Source: CAD feature listing. Evaluate the final solid. Frame: model axes, mm. A direction names the side the tool comes from. Coordinates: 2 decimals unless noted, no trailing zeros. Loops run counter-clockwise (first coordinate to the right, second up) from the corner with the lowest first, then second, coordinate; pieces in that order, holes last.
```python
from build123d import *

# Parameters (mm, degrees)
SKETCH1_R           = 23.8125
SKETCH1_R_2         = 10.4775
SKETCH1_R_3         = 1.905
BOSS_EXTRUDE1_DEPTH = 3.683


with BuildPart() as part:
    # Sketch1 → Boss-Extrude1 (new body)
    with BuildSketch(Plane(origin=(0, 0, 0), x_dir=(1, 0, 0), z_dir=(0, 1, 0))):
        with BuildLine():
            Line((-8.06473402, -4.72806869), (-8.06473402, 14.671308994))
            ThreePointArc((-8.06473402, 14.671308994), (-9.661605647, 23.535341917), (-14.251433206, 31.284829748))
            Line((-14.251433206, 31.284829748), (-39.858713959, 60.899286273))
            ThreePointArc((-39.858713959, 60.899286273), (-38.889761495, 87.184032671), (-12.602664438, 88.086967018))
            Line((-12.602664438, 88.086967018), (16.963304526, 62.391553913))
            ThreePointArc((16.963304526, 62.391553913), (24.731110608, 57.771090259), (33.625027761, 56.16306869))
            Line((33.625027761, 56.16306869), (53.14973402, 56.16306869))
            ThreePointArc((53.14973402, 56.16306869), (55.39479805, 55.23313272), (56.32473402, 52.98806869))
            Line((56.32473402, 52.98806869), (56.32473402, -4.72806869))
            ThreePointArc((56.32473402, -4.72806869), (55.39479805, -6.97313272), (53.14973402, -7.90306869))
            Line((53.14973402, -7.90306869), (-4.88973402, -7.90306869))
            ThreePointArc((-4.88973402, -7.90306869), (-7.13479805, -6.97313272), (-8.06473402, -4.72806869))
        make_face()
        with Locations(Location((24.13, 24.13, 0), (0, 0, 270))):
            Circle(SKETCH1_R, mode=Mode.SUBTRACT)
        with Locations(Location((-25.261408666, 73.521408666, 0), (0, 0, 270))):
            Circle(SKETCH1_R_2, mode=Mode.SUBTRACT)
        with Locations(Location((-36.294042469, 84.309426168, 0), (0, 0, 270))):
            Circle(SKETCH1_R_3, mode=Mode.SUBTRACT)
        with Locations(Location((-29.421941059, 88.38042278, 0), (0, 0, 270))):
            Circle(SKETCH1_R_3, mode=Mode.SUBTRACT)
        with Locations(Location((-10.402394551, 77.681941059, 0), (0, 0, 270))):
            Circle(SKETCH1_R_3, mode=Mode.SUBTRACT)
        with Locations(Location((-10.312858771, 69.695028354, 0), (0, 0, 270))):
            Circle(SKETCH1_R_3, mode=Mode.SUBTRACT)
        with Locations(Location((-29.087788977, 58.572858771, 0), (0, 0, 270))):
            Circle(SKETCH1_R_3, mode=Mode.SUBTRACT)
        with Locations(Location((-36.049426168, 62.488774863, 0), (0, 0, 270))):
            Circle(SKETCH1_R_3, mode=Mode.SUBTRACT)
        with BuildLine():
            ThreePointArc((44.60009114, -5.905215683), (49.831544821, -1.571544821), (54.165215683, 3.65990886))
            ThreePointArc((54.165215683, 3.65990886), (53.580347261, 6.748102738), (50.492153383, 6.163234317))
            ThreePointArc((50.492153383, 6.163234317), (46.688455179, 1.571544821), (42.096765683, -2.232153383))
            ThreePointArc((42.096765683, -2.232153383), (41.511897262, -5.320347261), (44.60009114, -5.905215683))
        make_face(mode=Mode.SUBTRACT)
        with BuildLine():
            ThreePointArc((44.60009114, 54.165215683), (49.831544821, 49.831544821), (54.165215683, 44.60009114))
            ThreePointArc((54.165215683, 44.60009114), (53.580347261, 41.511897262), (50.492153383, 42.096765683))
            ThreePointArc((50.492153383, 42.096765683), (46.688455179, 46.688455179), (42.096765683, 50.492153383))
            ThreePointArc((42.096765683, 50.492153383), (41.511897262, 53.580347261), (44.60009114, 54.165215683))
        make_face(mode=Mode.SUBTRACT)
        with BuildLine():
            ThreePointArc((3.65990886, -5.905215683), (-1.571544821, -1.571544821), (-5.905215683, 3.65990886))
            ThreePointArc((-5.905215683, 3.65990886), (-5.320347261, 6.748102738), (-2.232153383, 6.163234317))
            ThreePointArc((-2.232153383, 6.163234317), (1.571544821, 1.571544821), (6.163234317, -2.232153383))
            ThreePointArc((6.163234317, -2.232153383), (6.748102738, -5.320347261), (3.65990886, -5.905215683))
        make_face(mode=Mode.SUBTRACT)
        with BuildLine():
            ThreePointArc((3.65990886, 54.165215683), (-1.571544821, 49.831544821), (-5.905215683, 44.60009114))
            ThreePointArc((-5.905215683, 44.60009114), (-5.320347261, 41.511897262), (-2.232153383, 42.096765683))
            ThreePointArc((-2.232153383, 42.096765683), (1.571544821, 46.688455179), (6.163234317, 50.492153383))
            ThreePointArc((6.163234317, 50.492153383), (6.748102738, 53.580347261), (3.65990886, 54.165215683))
        make_face(mode=Mode.SUBTRACT)
    extrude(amount=BOSS_EXTRUDE1_DEPTH)


solid = part.part
```
Q1. First-contact query: pin 1 Ø1.5 at (y, z) = (2.5, -45) entering from -X; pin 2 Ø2.5 at (x, z) = (-10.4, -77.68) entering from +Y; pin 3 Ø1 at (y, z) = (1, -69.5) entering from -X; pin 4 Ø2 at (y, z) = (2.5, -64) entering from +X. Flat tips, straight axial feed; report the tip coordinate or a pass-through.
Q2. Section query C-C on y = 3.1. Count the separate pieces of the cut face and the enclosed holes in it, then the cut area to 3 significant figures.
Q3. Reachability of faces 1 (the cylindrical face through (49.764, 1.816, 1.639)), 2 (the cylindrical face through (55.42, 1.82, 6.95)), 3 (the flat face through (43, 2, -56.163)) from +Z, -Z, +X, -X, +Y, -Y: full face, straight path, thin tool, end or side. Return the list, or none.
Q4. Draft query along Z for faces 4 (the flat face through (-8.065, 2, -5)), 5 (the cylindrical face through (-35.7, 1.8, -82.5)), 6 (the cylindrical face through (-9.62, 1.82, -23.42)). Return one class per face: released by +Z, released by -Z, zero draft, split by the parting line, or undercut.
Q5. Material intervals for line 1 along X through (y, z) = (1.4, -77); line 2 along Z through (x, y) = (48.5, 1.4); line 3 along Z through (x, y) = (2.5, 2.15), sorted ascending.
Q6. Section query A-A on z = -24.13. Return the cut outline in (x, y), then the cut area to 3 significant figures.
Q7. Section query B-B on x = 24.13. Return the cut outline in (y, z).
Resolved:
1. pin 1: stops at x = -26.76
1. pin 2: passes through
1. pin 3: stops at x = -44.24
1. pin 4: stops at x = 16.26
2. separate pieces: 1
2. enclosed holes: 12
2. area: 3,710 mm2
3. face 1: +Y, -Y
3. face 2: +Z, +X, +Y, -Y
3. face 3: -Z, +X, +Y, -Y
4. face 4: zero draft
4. face 5: undercut
4. face 6: released by +Z
5. line 1: x = -44.24 to -35.14, -15.38 to -12.18, -8.62 to 0.15
5. line 2: z = -56.16 to -51.1, -44.72 to -3.54, 2.84 to 7.9
5. line 3: z = -74.96 to -53.34, -47.58 to -34.09, -14.17 to -0.68, 5.08 to 7.9
6. outline: (-9.89, 0) - (0.32, 0) - (0.32, 3.68) - (-9.89, 3.68) - close; (47.94, 0) - (56.32, 0) - (56.32, 3.68) - (47.94, 3.68) - close
6. area: 68.5 mm2
7. outline: (0, -58) - (3.68, -58) - (3.68, -47.94) - (0, -47.94) - close; (0, -0.32) - (3.68, -0.32) - (3.68, 7.9) - (0, 7.9) - close
